Input: dimensioned drawing with shaded views. Units: mm. Origin: part minimum x, y, z. A direction names the side the tool comes from. Round coordinates to 2 decimals unless told otherwise and drop trailing zeros. Loops run counter-clockwise (first coordinate to the right, second up) from the corner with the lowest first, then second, coordinate; pieces in that order, holes last. Notation, with made-up numbers: (36.25, 54) - (50.25, 54) arc R23 ccw to (50.25, 76) - close; hole circle Ø3 at (5, 31.5). An arc over 180 degrees is marked (long way). Answer as a JSON object with one key per item and string values. Group by question number.
Item 1: Line query: line 1 (X direction, y = 6.5, z = 33); line 2 (X direction, y = 7, z = 14). Output: solid intervals per line, ascending.
Item 2: First-contact query: pin 1 (4 mm diameter, centred on x = 44, y = 5, fed in from +Z); pin 2 (5 mm diameter, centred on y = 8, z = 12.5, fed in from -X). Flat tips, straight axial feed; report the tip coordinate or a pass-through.
Item 3: Section B-B (x = 34). Return the cut outline in (y, z).
Item 4: Section A-A (y = 6.75). Return the cut outline in (x, z), plus the area to 3 significant figures.
Item 5: Reachability of the marked faces 1, 2 and 3 from +Z, -Z, +X, -X, +Y, -Y: full face, straight path, thin tool, end or side. Return the list, or none.
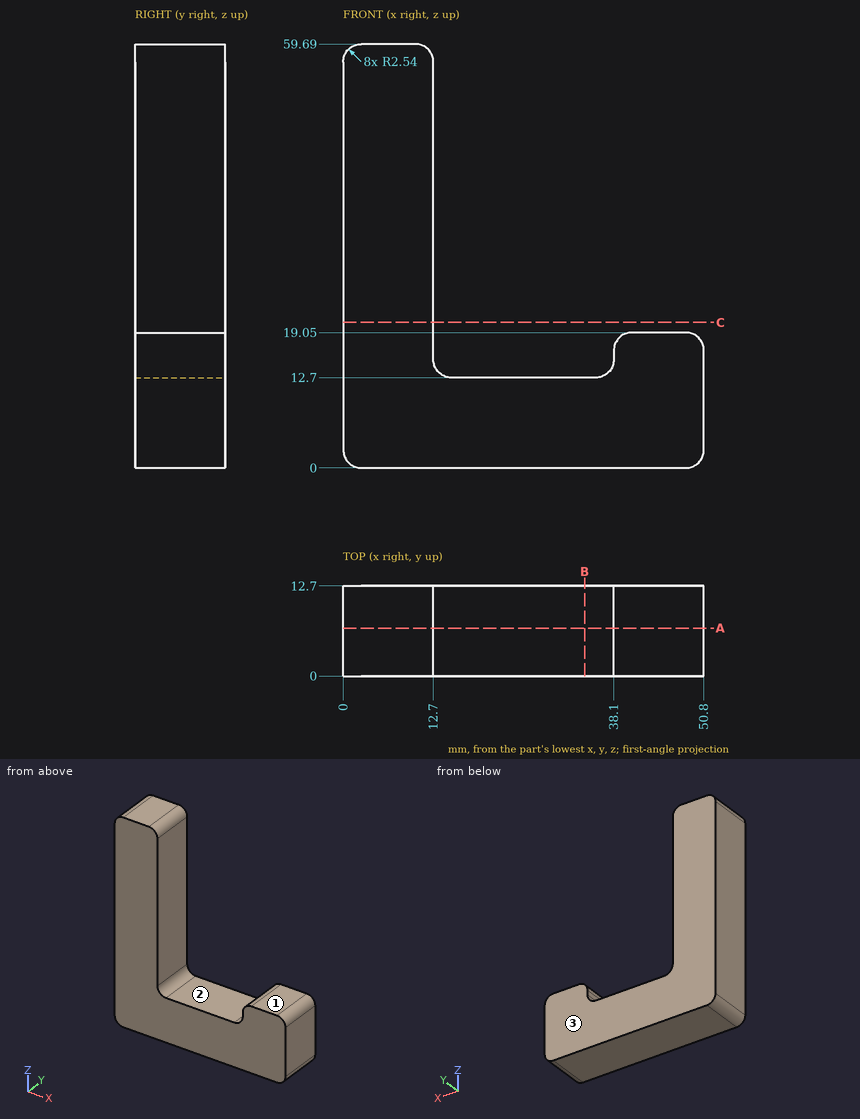
Values:
{
 "1": {"line 1": "x = 0 to 12.7", "line 2": "x = 0 to 13.02, 37.78 to 50.8"},
 "2": {"pin 1": "stops at z = 19.05", "pin 2": "stops at x = 0"},
 "3": {"outline": "(0, 0) - (12.7, 0) - (12.7, 12.7) - (0, 12.7) - close"},
 "4": {"outline": "(0, 2.54) arc R2.54 ccw to (2.54, 0) - (48.26, 0) arc R2.54 ccw to (50.8, 2.54) - (50.8, 16.51) arc R2.54 ccw to (48.26, 19.05) - (40.64, 19.05) arc R2.54 ccw to (38.1, 16.51) - (38.1, 15.24) arc R2.54 cw to (35.56, 12.7) - (15.24, 12.7) arc R2.54 cw to (12.7, 15.24) - (12.7, 57.15) arc R2.54 ccw to (10.16, 59.69) - (2.54, 59.69) arc R2.54 ccw to (0, 57.15) - close", "area": "1,320 mm^2"},
 "5": {"face 1": "+Z, +X, +Y, -Y", "face 2": "+Z, +Y, -Y", "face 3": "+Z, -Z, +X, -X, +Y"}
}
